Input: dimensioned drawing with shaded views. Units: mm. Origin: part minimum x, y, z. A direction names the side the tool comes from. Coordinates: 2 decimals unless noted, no trailing zeros. Loops run counter-clockwise (first coordinate to the right, second up) from the corner with the lowest first, then second, coordinate; pieces in that order, holes last.
Item 1: Ray query, line 1 along Z through (x, y) = (104, 75); line 2 along X through (y, z) = (76.5, 69.8); line 3 along X through (y, z) = (78, 69). Return the intervals inside material, ascending.
Item 2: Section D-D on x = 58. Return loops of the section in (y, z).
Item 3: Section B-B on y = 24. Return loops of the section in (x, z), and give its area (3 significant figures).
Item 4: Section A-A on z = 69.8. Return loops of the section in (x, y), and give its area (3 significant figures).
Item 5: Reachability of the marked faces 1 and 2 from +Z, -Z, +X, -X, +Y, -Y: full face, straight path, thin tool, end or side. Return the list, or none.
Item 6: Contact query for flat-ended pins moving along their axis: P1, Ø21.5, axis at x = 83.5, y = 52.5, coming from the +Z side; P2, Ø6, axis at x = 97.5, y = 29.5, coming from the +Z side. Output: stop coordinate, or through.
Item 7: Section C-C on x = 104. Return loops of the section in (y, z).
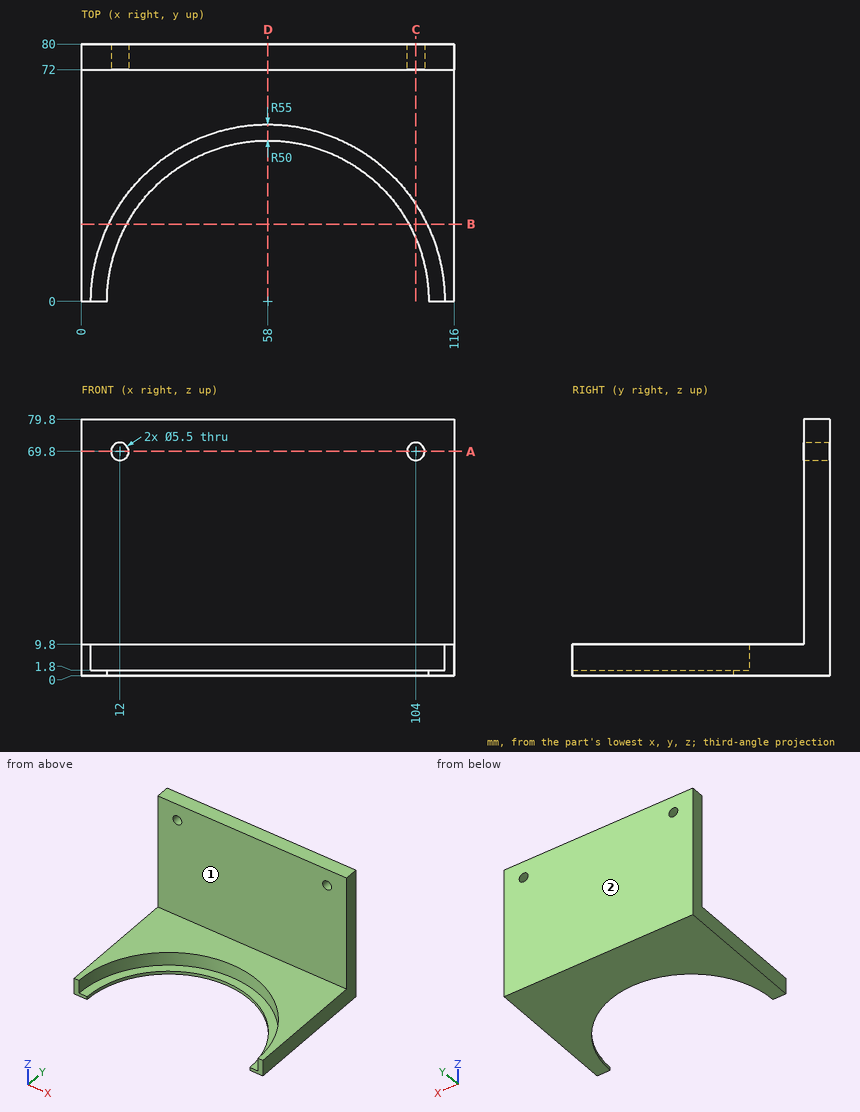
Results found:
1. line 1: z = 0 to 67.05, 72.55 to 79.8
1. line 2: x = 0 to 9.25, 14.75 to 101.25, 106.75 to 116
1. line 3: x = 0 to 9.37, 14.63 to 101.37, 106.63 to 116
2. outline: (50, 0) - (80, 0) - (80, 79.8) - (72, 79.8) - (72, 9.8) - (55, 9.8) - (55, 1.8) - (50, 1.8) - close
3. outline: (0, 0) - (14.14, 0) - (14.14, 1.8) - (8.51, 1.8) - (8.51, 9.8) - (0, 9.8) - close; (101.86, 0) - (116, 0) - (116, 9.8) - (107.49, 9.8) - (107.49, 1.8) - (101.86, 1.8) - close
3. area: 187 mm2
4. outline: (0, 72) - (9.25, 72) - (9.25, 80) - (0, 80) - close; (14.75, 72) - (101.25, 72) - (101.25, 80) - (14.75, 80) - close; (106.75, 72) - (116, 72) - (116, 80) - (106.75, 80) - close
4. area: 840 mm2
5. face 1: +Z, +X, -X, -Y
5. face 2: +Z, -Z, +X, -X, +Y
6. P1: stops at z = 9.8
6. P2: stops at z = 1.8
7. outline: (19.6, 0) - (80, 0) - (80, 67.05) - (72, 67.05) - (72, 9.8) - (30.15, 9.8) - (30.15, 1.8) - (19.6, 1.8) - close; (72, 72.55) - (80, 72.55) - (80, 79.8) - (72, 79.8) - close
